```python
from build123d import *

# Parameters (mm, degrees)
F0_R     = 3.1
F1_DEPTH = 10
F2_DEPTH = 1
F3_W     = 5
F3_H     = 1
F4_DEPTH = 11.001


# Not quite as in the source:
# - a feature names something its author has since deleted; it is built from what else it names


with BuildPart() as f1:
    # F0 (on Top) → F1 (new body, symmetric)
    with BuildSketch(Plane.XY):
        Circle(F0_R)
    extrude(amount=F1_DEPTH, both=True)

    # F0 (on Top) → F2 (join, symmetric)
    with BuildSketch(Plane.XY):
        with BuildLine():
            ThreePointArc((1.6906573106, -9.8560477808), (7.645474907, -6.4456740103), (10, 0))
            ThreePointArc((10, 0), (7.6454749578, 6.44567395), (1.6906574661, 9.8560477542))
            ThreePointArc((1.6906574661, 9.8560477542), (-10, 7.89e-08), (1.6906573106, -9.8560477808))
        make_face()
        Circle(F0_R, mode=Mode.SUBTRACT)
        with BuildLine():
            ThreePointArc((1.6906574661, 9.8560477542), (7.6454749578, 6.44567395), (10, 0))
            ThreePointArc((10, 0), (7.645474907, -6.4456740103), (1.6906573106, -9.8560477808))
            Line((1.6906573106, -9.8560477808), (30, -5))
            Line((30, -5), (30, 5))
            Line((30, 5), (1.6906574661, 9.8560477542))
        make_face()
    extrude(amount=F2_DEPTH, both=True)

    # F3 (on face) → F4 (cut, through all)
    with BuildSketch(Plane.XY.offset(1)):
        with Locations((27.5, 0)):
            Rectangle(F3_W, F3_H)
    extrude(amount=-F4_DEPTH, mode=Mode.SUBTRACT)


solid = f1.part
```
Geometry check sheet. Reference: the model listing, model coordinates, mm. A direction names the side the tool comes from. Give positions to 0.01 mm unless a question says otherwise; leave off trailing zeros. Loops run counter-clockwise (first coordinate to the right, second up) from the corner with the lowest first, then second, coordinate; pieces in that order, holes last. Notation, with made-up numbers: (53.25, 39) - (75.25, 39) arc R15 cw to (75.25, 44) - close; hole circle Ø10 at (46.25, 79.5). An arc over 180 degrees is marked (long way). Use CSV: the item, a comma, the result in double quotes. Start each with the question number.
Q1. Section check A-A, the plane y = 0. Record the cut outline in (x, z).
Q2. Section check B-B, the plane x = 0. Record the cut outline in (y, z), and give its area (3 significant figures).
Q3. Section check C-C, the plane z = -7.25. Record the cut outline in (x, y), and give its area (3 significant figures).
Q4. Go/stop test with flat-tipped pins: pin 1 Ø1 at (y, z) = (2.5, -2.5) entering from -X; pin 2 Ø2 at (x, z) = (24, 1.5) entering from -Y; pin 3 Ø1 at (x, z) = (28, 0) entering from -Y. Record where each tip stops, or that it passes through.
Q5. Scan lines: probe 1 along Z at (x, y) = (-3, 3.5); probe 2 along X at (y, z) = (-0.25, 6.75); probe 3 along Y at (x, z) = (1, -7). Record each from-to range of solid material in increasing order. Write a range as from..to.
Q6. Section check D-D, the plane y = -7.75. Record the cut outline in (x, z), and give its area (3 significant figures).
Q7. Access from +Z, -Z, +X, -X, +Y, -Y to the whole of each face (thin tool, end or side, straight path). Record for faces 1 (the face through (1.43, -2.75, 5.56)), 2 (the face through (27, 0.5, 0)), 3 (the face through (1.43, -2.75, -5.44)).
Findings below:
1,outline,"(-10, -1) - (-3.1, -1) - (-3.1, -10) - (3.1, -10) - (3.1, -1) - (25, -1) - (25, 1) - (3.1, 1) - (3.1, 10) - (-3.1, 10) - (-3.1, 1) - (-10, 1) - close"
2,outline,"(-10, -1) - (-3.1, -1) - (-3.1, -10) - (3.1, -10) - (3.1, -1) - (10, -1) - (10, 1) - (3.1, 1) - (3.1, 10) - (-3.1, 10) - (-3.1, 1) - (-10, 1) - close"
2,area,"152 mm^2"
3,outline,"circle Ø6.2 at (0, 0)"
3,area,"30.2 mm^2"
4,pin 1,"stops at x = -2.37"
4,pin 2,"stops at y = -6.18"
4,pin 3,"stops at y = -5.43"
5,probe 1,"z = -1..1"
5,probe 2,"x = -3.09..3.09"
5,probe 3,"y = -2.93..2.93"
6,outline,"(-6.32, -1) - (13.97, -1) - (13.97, 1) - (-6.32, 1) - close"
6,area,"40.6 mm^2"
7,face 1,"+Z"
7,face 2,"+Z, -Z, +X"
7,face 3,"-Z"
